Build history of the part. All positions in model axes, mm. A direction names the side the tool comes from. Round coordinates to 2 decimals unless told otherwise and drop trailing zeros. Write each loop counter-clockwise with the first axis right and the second up, starting at its lowest first coordinate (ties: lowest second). Pieces come first, ordered by that corner, then holes. Notation, with made-up numbers: M 48.5,41.5 L 57.5,41.5 A15 cw 57.5,54.5 Z; hole C 56,-11.75 d7. An arc over 180 degrees is marked long. Use a Markdown table: item, result.
from build123d import *

# Parameters (mm, degrees)
SKETCH2_R           = 17.5
SKETCH2_R_2         = 9.2
BOSS_EXTRUDE1_DEPTH = 2.5
BOSS_EXTRUDE2_START = -0.6
SKETCH3_R           = 9.2
SKETCH3_R_2         = 7.5
BOSS_EXTRUDE2_DEPTH = 0.6
SKETCH4_R           = 1.67
CUT_EXTRUDE1_DEPTH  = 1.15
CIRPATTERN1_COUNT   = 4


with BuildPart() as part:
    # Sketch2 → Boss-Extrude1 (new body)
    with BuildSketch(Plane(origin=(0, 0, 0), x_dir=(1, 0, 0), z_dir=(0, 1, 0))):
        with Locations(Location((-21.383734207, -0.621346489, 0), (0, 0, 270))):
            Circle(SKETCH2_R)
        with Locations(Location((-21.383734207, -0.621346489, 0), (0, 0, 270))):
            Circle(SKETCH2_R_2, mode=Mode.SUBTRACT)
    extrude(amount=BOSS_EXTRUDE1_DEPTH)

    # Sketch3 → Boss-Extrude2 (add)
    with BuildSketch(Plane(origin=(0, 2.5, 0), x_dir=(1, 0, 0), z_dir=(0, 1, 0)).offset(BOSS_EXTRUDE2_START)):
        with Locations(Location((-21.383734207, -0.621346489, 0), (0, 0, 270))):
            Circle(SKETCH3_R)
        with Locations(Location((-21.383734207, -0.621346489, 0), (0, 0, 270))):
            Circle(SKETCH3_R_2, mode=Mode.SUBTRACT)
    extrude(amount=BOSS_EXTRUDE2_DEPTH)

    # Sketch4 → Cut-Extrude1 (cut)
    with BuildSketch(Plane.XZ):
        with Locations(Location((-21.569675845, 15.589648339, 0), (0, 0, 270))):
            Circle(SKETCH4_R)
    cut_extrude1 = extrude(amount=-CUT_EXTRUDE1_DEPTH, mode=Mode.SUBTRACT)

    # CirPattern1: Cut-Extrude1 ×4 about axis
    cirpattern1_axis = Axis((-21.383734207, 0, 0.621346489), (0, 1, 0))
    for i in range(1, CIRPATTERN1_COUNT):
        add(cut_extrude1.rotate(cirpattern1_axis, i * 360 / CIRPATTERN1_COUNT), mode=Mode.SUBTRACT)


solid = part.part
Q1. Drill centre lines: L1, parallel to Z at x = -22.5, y = 0.55; L2, parallel to X at y = 0.75, z = 15.5; L3, parallel to X at y = 0.3, z = -4.5. Where is each one in solid material? Low to high.
Response values:
| item | result |
|---|---|
| L1 | z = -16.84 to -15.39, -13.3 to -8.51, 9.75 to 14.2, 16.98 to 18.09 |
| L2 | x = -30.6 to -23.24, -19.9 to -12.17 |
| L3 | x = -38.12 to -29.03, -13.74 to -4.65 |
Q2. Two-plate mould, pull along X, no slides. Class faces 3 (the cylindrical face through (-5.185, 0.567, -0.321)), 4 (the flat face through (-25, 2.5, 8)), 5 (the cylindrical face through (-38.47, 1.23, -3.17)): +X half, -X half, draft (parallel to the pull), parting line (faces both ways), or undercut.
Response values:
| item | result |
|---|---|
| face 3 | undercut |
| face 4 | draft |
| face 5 | parting line |
Q3. Cut at C-C on x = -11. Give the cut face in (y, z).
Response values:
| item | result |
|---|---|
| outline | M 0,-13.47 L 2.5,-13.47 L 2.5,14.71 L 0,14.71 Z |
Q4. Cut at B-B on x = -17.5. Give the cut face in (y, z), and give its area (3 significant figures).
Response values:
| item | result |
|---|---|
| outline | M 0,-16.44 L 2.5,-16.44 L 2.5,-5.79 L 1.9,-5.79 L 1.9,-7.72 L 0,-7.72 Z; M 0,8.96 L 1.9,8.96 L 1.9,7.04 L 2.5,7.04 L 2.5,17.68 L 0,17.68 Z |
| area | 45.9 mm2 |
Q5. Drop flat-ended pins along their axis: P1, Ø17, axis at x = -21.38, z = 0.62, coming from the -Y side; P2, Ø2.5, axis at x = -21, z = 15.5, coming from the -Y side; P3, Ø1.7, axis at x = -6.5, z = 1, coming from the -Y side; P4, Ø1, axis at y = 1.5, z = 5, coming from the +X side. Give the stop position or say it passes through.
Response values:
| item | result |
|---|---|
| P1 | stops at y = 1.9 |
| P2 | stops at y = 0 |
| P3 | stops at y = 1.15 |
| P4 | stops at x = -4.32 |
Q6. Cut at D-D on x = -31. Give the cut face in (y, z), and give its area (3 significant figures).
Response values:
| item | result |
|---|---|
| outline | M 0,-14 L 2.5,-14 L 2.5,15.24 L 0,15.24 Z |
| area | 73.1 mm2 |
Q7. Which spindle directions (+Z, -Z, +X, -X, +Y, -Y) get a long thin tool onto all of the face, cutting with end or side? Do faces 1 (the flat face through (-36, 1.15, 0)), 2 (the flat face through (-29, 0, 8)). Say none if no direction does.
Response values:
| item | result |
|---|---|
| face 1 | -Y |
| face 2 | +Z, -Z, +X, -X, -Y |
Q8. Cut at A-A on z = 6.5. Give the cut face in (x, y).
Response values:
| item | result |
|---|---|
| outline | M -37.87,0 L -28.46,0 L -28.46,1.9 L -26.04,1.9 L -26.04,2.5 L -37.87,2.5 Z; M -16.73,1.9 L -14.31,1.9 L -14.31,0 L -4.9,0 L -4.9,2.5 L -16.73,2.5 Z |
